CAD build for the part. Positions are in the model's coordinates, mm. Face numbers are marked on the shaded views. A direction names the side the tool comes from. Round coordinates to 2 decimals unless told otherwise and drop trailing zeros. Write each loop counter-clockwise with the first axis right and the second up, starting at its lowest first coordinate (ties: lowest second). Pieces come first, ordered by that corner, then holes. Notation, with made-up numbers: (24, -6) - (55, -6) arc R24 cw to (55, 24) - close; hole circle Ø9 at (-21, 28). An arc over 180 degrees is marked (long way). Answer in a Markdown table with one row per item.
```python
from build123d import *

# Parameters (mm, degrees)
SKETCH1_R           = 2.15
BOSS_EXTRUDE1_DEPTH = 10
SKETCH3_W           = 75
SKETCH3_H           = 3
CUT_EXTRUDE1_DEPTH  = 4
SKETCH4_W           = 40
SKETCH4_H           = 25
CUT_EXTRUDE2_DEPTH  = 44.660622991
SKETCH5_R           = 1
CUT_EXTRUDE3_DEPTH  = 44.660622991


with BuildPart() as part:
    # Sketch1 → Boss-Extrude1 (new body)
    with BuildSketch(Plane.XY):
        Polygon((21, 5), (37.5, 5), (37.5, -20), (-37.5, -20), (-37.5, 5), (-21, 5), (-21, -10), (21, -10), align=None)
        with Locations((-30.5, 0)):
            Circle(SKETCH1_R, mode=Mode.SUBTRACT)
        with Locations((-30.5, -12)):
            Circle(SKETCH1_R, mode=Mode.SUBTRACT)
        with Locations((30.5, 0)):
            Circle(SKETCH1_R, mode=Mode.SUBTRACT)
        with Locations((30.5, -12)):
            Circle(SKETCH1_R, mode=Mode.SUBTRACT)
    extrude(amount=BOSS_EXTRUDE1_DEPTH)

    # Sketch3 → Cut-Extrude1 (cut)
    with BuildSketch(Plane(origin=(0, 0, 0), x_dir=(-1, 0, 0), z_dir=(0, 0, -1))):
        with Locations((0, -18.5)):
            Rectangle(SKETCH3_W, SKETCH3_H)
    extrude(amount=-CUT_EXTRUDE1_DEPTH, mode=Mode.SUBTRACT)

    # Sketch4 → Cut-Extrude2 (cut, through all)
    with BuildSketch(Plane.XY.offset(10)):
        with Locations((17.5, -7.5)):
            Rectangle(SKETCH4_W, SKETCH4_H)
    extrude(amount=-CUT_EXTRUDE2_DEPTH, mode=Mode.SUBTRACT)

    # Sketch5 → Cut-Extrude3 (cut, through all)
    with BuildSketch(Plane.XY.offset(10)):
        with Locations((-7.5, -14)):
            Circle(SKETCH5_R)
        with Locations((-17, -14)):
            Circle(SKETCH5_R)
    extrude(amount=-CUT_EXTRUDE3_DEPTH, mode=Mode.SUBTRACT)


solid = part.part
```
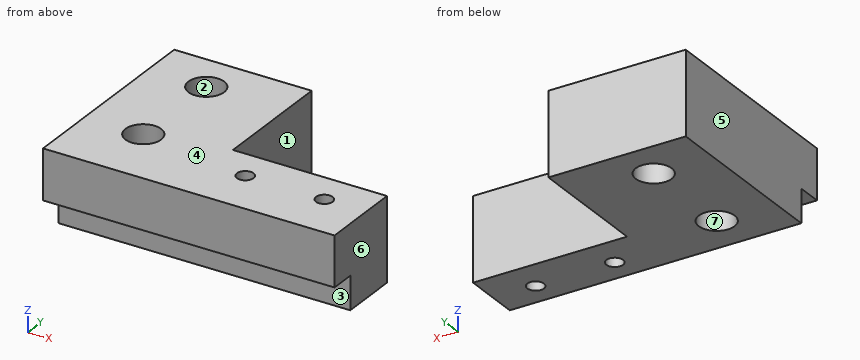
Q1. Flat gauge pins, fed straight in: pin 1 (2 mm diameter, centred on x = -23, z = 2, fed in from -Y); pin 2 (3 mm diameter, centred on y = -3.5, z = 4.5, fed in from +X); pin 3 (5 mm diameter, centred on x = -15, z = 7, fed in from +Y); pin 4 (1.8 mm diameter, centred on x = -7.5, y = -14, fed in from +Z). Where does each tip first touch, or does it go through?
Computed:
| item | result |
|---|---|
| pin 1 | stops at y = -17 |
| pin 2 | stops at x = -21 |
| pin 3 | stops at y = -10 |
| pin 4 | passes through |
Q2. Saw through at A-A on y = -12. List the corners of the cut face in (x, z), then the cut area to 3 significant figures.
Computed:
| item | result |
|---|---|
| outline | (-37.5, 0) - (-32.65, 0) - (-32.65, 10) - (-37.5, 10) - close; (-28.35, 0) - (-2.5, 0) - (-2.5, 10) - (-28.35, 10) - close |
| area | 307 mm2 |
Q3. Saw through at D-D on z = 3.25. List the corners of the cut face in (x, y).
Computed:
| item | result |
|---|---|
| outline | (-37.5, -17) - (-2.5, -17) - (-2.5, -10) - (-21, -10) - (-21, 5) - (-37.5, 5) - close; hole circle Ø4.3 at (-30.5, -12); hole circle Ø4.3 at (-30.5, 0); hole circle Ø2 at (-17, -14); hole circle Ø2 at (-7.5, -14) |
Q4. Saw through at C-C on x = -17. List the corners of the cut face in (y, z).
Computed:
| item | result |
|---|---|
| outline | (-20, 4) - (-17, 4) - (-17, 0) - (-15, 0) - (-15, 10) - (-20, 10) - close; (-13, 0) - (-10, 0) - (-10, 10) - (-13, 10) - close |
Q5. Pull direction X, two halves, no side cores. Call the marked faces 4, 5, 6 and 7: released by +X, released by -X, zero draft, split by the parting line, or undercut.
Computed:
| item | result |
|---|---|
| face 4 | zero draft |
| face 5 | released by -X |
| face 6 | released by +X |
| face 7 | undercut |
Q6. 3-axis set-ups, long thin cutter, end or side, ignore diameter. For the marked faces 1, 2 and 3: which of +Z, -Z, +X, -X, +Y, -Y reach the whole face in a straight line?
Computed:
| item | result |
|---|---|
| face 1 | +Z, -Z, +X, +Y |
| face 2 | +Z, -Z |
| face 3 | -Z, +X, -X, -Y |
Q7. Saw through at B-B on z = 7.5. List the corners of the cut face in (x, y), then the cut area to 3 significant figures.
Computed:
| item | result |
|---|---|
| outline | (-37.5, -20) - (-2.5, -20) - (-2.5, -10) - (-21, -10) - (-21, 5) - (-37.5, 5) - close; hole circle Ø4.3 at (-30.5, -12); hole circle Ø4.3 at (-30.5, 0); hole circle Ø2 at (-17, -14); hole circle Ø2 at (-7.5, -14) |
| area | 562 mm2 |
Q8. Drill centre lines: line 1 (Y direction, x = -30.5, z = 3); line 2 (Y direction, x = -7.5, z = 1); line 3 (Y direction, x = -7.5, z = 6). Where is each one in solid material? Low to high.
Computed:
| item | result |
|---|---|
| line 1 | y = -17 to -14.15, -9.85 to -2.15, 2.15 to 5 |
| line 2 | y = -17 to -15, -13 to -10 |
| line 3 | y = -20 to -15, -13 to -10 |
